Check sheet for the modelled part. Datum: model origin and axes. Units: mm. A direction names the side the tool comes from. Coordinates: 2 decimals unless noted, no trailing zeros. Loops run counter-clockwise (first coordinate to the right, second up) from the corner with the lowest first, then second, coordinate; pieces in that order, holes last.
from build123d import *

# Parameters (mm, degrees)
BOSS_EXTRUDE1_DEPTH = 5
SKETCH3_R           = 2
CUT_EXTRUDE1_DEPTH  = 5
SKETCH4_R           = 11
CUT_EXTRUDE2_DEPTH  = 10


with BuildPart() as part:
    # Sketch2 → Boss-Extrude1 (new body)
    with BuildSketch(Plane.XY):
        with BuildLine():
            Line((-15.357210304, 0), (-22.5, 0))
            Line((-22.5, 0), (-2.5, -22.360679775))
            ThreePointArc((-2.5, -22.360679775), (0, -22.5), (2.5, -22.360679775))
            Line((2.5, -22.360679775), (22.5, 0))
            Line((22.5, 0), (15.357210304, 0))
            ThreePointArc((15.357210304, 0), (0, -6.055970942), (-15.357210304, 0))
        make_face()
        with BuildLine():
            ThreePointArc((-2.5, -22.360679775), (-16.770509831, -15), (-22.5, 0))
            Line((-22.5, 0), (-44.860679775, -20))
            Line((-44.860679775, -20), (-24.860679775, -42.360679775))
            Line((-24.860679775, -42.360679775), (-2.5, -22.360679775))
        make_face()
        with BuildLine():
            ThreePointArc((-20.943936523, 8.222014529), (-22.107561735, 4.183983044), (-22.5, 0))
            Line((-22.5, 0), (-15.357210304, 0))
            ThreePointArc((-15.357210304, 0), (-18.61031155, 3.798622619), (-20.943936523, 8.222014529))
        make_face()
        with BuildLine():
            Line((-2.5, -22.360679775), (-22.5, 0))
            ThreePointArc((-22.5, 0), (-16.770509831, -15), (-2.5, -22.360679775))
        make_face()
        with BuildLine():
            Line((-22.5, 16.444029058), (-22.5, 0))
            ThreePointArc((-22.5, 0), (-22.107561735, 4.183983044), (-20.943936523, 8.222014529))
            ThreePointArc((-20.943936523, 8.222014529), (-22.107561735, 12.260046014), (-22.5, 16.444029058))
        make_face()
        with BuildLine():
            ThreePointArc((22.5, 16.444029058), (0, 38.944029058), (-22.5, 16.444029058))
            Line((-22.5, 16.444029058), (-15.357210304, 16.444029058))
            ThreePointArc((-15.357210304, 16.444029058), (0, 22.5), (15.357210304, 16.444029058))
            Line((15.357210304, 16.444029058), (22.5, 16.444029058))
        make_face()
        with BuildLine():
            Line((-15.357210304, 16.444029058), (-22.5, 16.444029058))
            ThreePointArc((-22.5, 16.444029058), (-22.107561735, 12.260046014), (-20.943936523, 8.222014529))
            ThreePointArc((-20.943936523, 8.222014529), (-18.61031155, 12.64540644), (-15.357210304, 16.444029058))
        make_face()
        with BuildLine():
            ThreePointArc((-20.943936523, 8.222014529), (-18.61031155, 3.798622619), (-15.357210304, 0))
            Line((-15.357210304, 0), (15.357210304, 0))
            ThreePointArc((15.357210304, 0), (18.61031155, 3.798622619), (20.943936523, 8.222014529))
            ThreePointArc((20.943936523, 8.222014529), (18.61031155, 12.64540644), (15.357210304, 16.444029058))
            Line((15.357210304, 16.444029058), (-15.357210304, 16.444029058))
            ThreePointArc((-15.357210304, 16.444029058), (-18.61031155, 12.64540644), (-20.943936523, 8.222014529))
        make_face()
        with BuildLine():
            Line((15.357210304, 0), (-15.357210304, 0))
            ThreePointArc((-15.357210304, 0), (0, -6.055970942), (15.357210304, 0))
        make_face()
        with BuildLine():
            ThreePointArc((22.5, 0), (16.770509831, -15), (2.5, -22.360679775))
            Line((2.5, -22.360679775), (24.860679775, -42.360679775))
            Line((24.860679775, -42.360679775), (44.860679775, -20))
            Line((44.860679775, -20), (22.5, 0))
        make_face()
        with BuildLine():
            Line((22.5, 0), (2.5, -22.360679775))
            ThreePointArc((2.5, -22.360679775), (16.770509831, -15), (22.5, 0))
        make_face()
        with BuildLine():
            ThreePointArc((15.357210304, 16.444029058), (0, 22.5), (-15.357210304, 16.444029058))
            Line((-15.357210304, 16.444029058), (15.357210304, 16.444029058))
        make_face()
        with BuildLine():
            ThreePointArc((20.943936523, 8.222014529), (22.107561735, 12.260046014), (22.5, 16.444029058))
            Line((22.5, 16.444029058), (15.357210304, 16.444029058))
            ThreePointArc((15.357210304, 16.444029058), (18.61031155, 12.64540644), (20.943936523, 8.222014529))
        make_face()
        with BuildLine():
            Line((22.5, 0), (22.5, 16.444029058))
            ThreePointArc((22.5, 16.444029058), (22.107561735, 12.260046014), (20.943936523, 8.222014529))
            ThreePointArc((20.943936523, 8.222014529), (22.107561735, 4.183983044), (22.5, 0))
        make_face()
        with BuildLine():
            ThreePointArc((20.943936523, 8.222014529), (18.61031155, 3.798622619), (15.357210304, 0))
            Line((15.357210304, 0), (22.5, 0))
            ThreePointArc((22.5, 0), (22.107561735, 4.183983044), (20.943936523, 8.222014529))
        make_face()
    extrude(amount=BOSS_EXTRUDE1_DEPTH)

    # Sketch3 → Cut-Extrude1 (cut)
    with BuildSketch(Plane(origin=(0, 0, 0), x_dir=(-1, 0, 0), z_dir=(0, 0, -1))):
        with Locations(Location((-37.800566479, -20.393446629, 0), (0, 0, 180))):
            Circle(SKETCH3_R)
        with Locations(Location((-22.893446629, -7.060113296, 0), (0, 0, 180))):
            Circle(SKETCH3_R)
        with Locations(Location((-9.560113296, -21.967233146, 0), (0, 0, 180))):
            Circle(SKETCH3_R)
        with Locations(Location((-24.467233146, -35.300566479, 0), (0, 0, 180))):
            Circle(SKETCH3_R)
        with Locations(Location((24.467233146, -35.300566479, 0), (0, 0, 180))):
            Circle(SKETCH3_R)
        with Locations(Location((37.800566479, -20.393446629, 0), (0, 0, 180))):
            Circle(SKETCH3_R)
        with Locations(Location((9.560113296, -21.967233146, 0), (0, 0, 180))):
            Circle(SKETCH3_R)
        with Locations(Location((22.893446629, -7.060113296, 0), (0, 0, 180))):
            Circle(SKETCH3_R)
    extrude(amount=-CUT_EXTRUDE1_DEPTH, mode=Mode.SUBTRACT)

    # Sketch4 → Cut-Extrude2 (cut)
    with BuildSketch(Plane(origin=(0, 0, 0), x_dir=(-1, 0, 0), z_dir=(0, 0, -1))):
        with Locations((0, 10)):
            Circle(SKETCH4_R)
    extrude(amount=-CUT_EXTRUDE2_DEPTH, mode=Mode.SUBTRACT)


solid = part.part
(1) Section check B-B, the plane x = 0. Enter the section's corners in (y, z).
(2) Set-up check for faces 4 (the face through (-22.5, 8, 2)), 5 (the face through (-0.63, -1.14, 0)), 6 (the face through (-13.837, -32.501, 2.465)): record each of +Z, -Z, +X, -X, +Y, -Y from which the full face is reachable in a straight line by a thin tool's end or side.
(3) Section check D-D, the plane y = 22. Enter the section's corners in (x, z), plus the area to 3 significant figures.
(4) Scan lines: line 1 along X through (y, z) = (-21.5, 1.95); line 2 along Y through (x, z) = (25, 3.4); line 3 along Y through (x, z) = (8, 1.95). Record each from-to range of solid material in increasing order.
(5) Draft check along X on faces 1 (the face through (-35.001, -31.024, 2.465)), 2 (the face through (33.837, -10.14, 2.465)), 3 (the face through (13.5, -32.2, 2.5)). Enter one of: pulls with the +X half, pulls with the -X half, needs draft (parallel to the pull), parting line crosses it, or undercut.
(6) Section check A-A, the plane y = 10. Enter the section's corners in (x, z).
(7) Gauge pin test, flat ends, axial feed: P1, Ø3, axis at x = 33.5, z = 3, coming from the -Y side; P2, Ø2.5, axis at x = -24.47, y = -35.3, coming from the +Z side; P3, Ø2.5, axis at y = 7.5, z = 2, coming from the +X side; P4, Ø2, axis at y = 25.5, z = 0.5, coming from the +X side. Record the tip position at first contact, or that the pin passes through.
(8) Section check C-C, the plane z = 1.6. Count the separate pieces of the cut face and the enclosed holes in it, plus the area to 3 significant figures.
Determined:
1. outline: (-22.5, 0) - (-1, 0) - (-1, 5) - (-22.5, 5) - close; (21, 0) - (38.94, 0) - (38.94, 5) - (21, 5) - close
2. face 4: +Z, -Z, -X, +Y
2. face 5: -Z, +X, -X, +Y, -Y
2. face 6: +Z, -Z, -Y
3. outline: (-21.8, 0) - (21.8, 0) - (21.8, 5) - (-21.8, 5) - close
3. area: 218 mm2
4. line 1: x = -43.52 to -39.47, -36.13 to -11.5, -7.62 to 7.62, 11.5 to 36.13, 39.47 to 43.52
4. line 2: y = -42.2 to -37.23, -33.37 to -2.24
4. line 3: y = -27.28 to -23.22, -20.72 to 2.45, 17.55 to 37.47
5. face 1: pulls with the -X half
5. face 2: pulls with the +X half
5. face 3: undercut
6. outline: (-22.5, 0) - (-11, 0) - (-11, 5) - (-22.5, 5) - close; (11, 0) - (22.5, 0) - (22.5, 5) - (11, 5) - close
7. P1: stops at y = -34.38
7. P2: passes through
7. P3: stops at x = 22.5
7. P4: stops at x = 21.01
8. separate pieces: 1
8. enclosed holes: 9
8. area: 3,410 mm2
